Design review of the part built by this model. Coordinates are the model's own, in mm. Give positions to 0.01 mm unless a question says otherwise; leave off trailing zeros. Loops run counter-clockwise (first coordinate to the right, second up) from the corner with the lowest first, then second, coordinate; pieces in that order, holes last. Notation, with made-up numbers: (28.5, 55) - (69.5, 55) arc R8 cw to (69.5, 69) - close; hole circle Ø10 at (3, 44.25). An arc over 180 degrees is marked (long way). One line per item, written item: value. Start each with the question number.
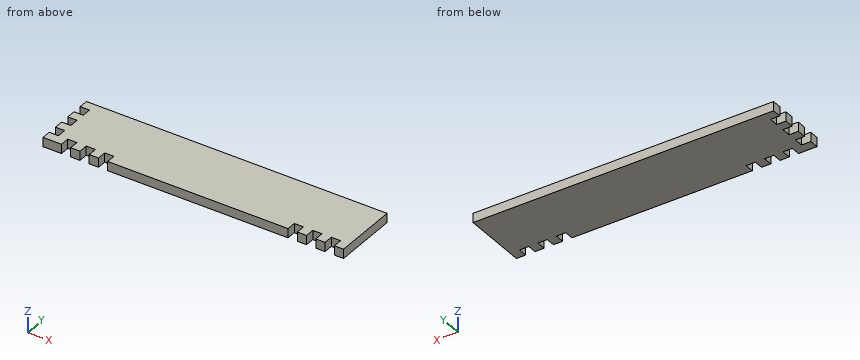
```python
from build123d import *

# Parameters (mm, degrees)
F0_W     = 412.75
F0_H     = 88.9
F1_DEPTH = 12.7
F2_W     = 12.7
F2_H     = 12.7
F3_DEPTH = 25.4
F4_W     = 12.7
F4_H     = 12.7
F5_DEPTH = 25.4
F6_W     = 12.7
F6_H     = 12.7
F7_DEPTH = 25.4


with BuildPart() as f1:
    # F0 (on Top) → F1 (new body)
    with BuildSketch(Plane.XY):
        with Locations((206.375, 44.45)):
            Rectangle(F0_W, F0_H)
    extrude(amount=F1_DEPTH)

    # F2 (on face) → F3 (cut)
    with BuildSketch(Plane.XY.offset(12.7)):
        with Locations((6.35, 19.05)):
            Rectangle(F2_W, F2_H)
        with Locations((6.35, 69.85)):
            Rectangle(F2_W, F2_H)
        with Locations((6.35, 44.45)):
            Rectangle(F2_W, F2_H)
    extrude(amount=-F3_DEPTH, mode=Mode.SUBTRACT)

    # F4 (on face) → F5 (cut)
    with BuildSketch(Plane.XY.offset(12.7)):
        with Locations((393.7, 6.35)):
            Rectangle(F4_W, F4_H)
        with Locations((368.3, 6.35)):
            Rectangle(F4_W, F4_H)
        with Locations((342.9, 6.35)):
            Rectangle(F4_W, F4_H)
    extrude(amount=-F5_DEPTH, mode=Mode.SUBTRACT)

    # F6 (on face) → F7 (cut)
    with BuildSketch(Plane.XY.offset(12.7)):
        with Locations((31.75, 6.35)):
            Rectangle(F6_W, F6_H)
        with Locations((57.15, 6.35)):
            Rectangle(F6_W, F6_H)
        with Locations((82.55, 6.35)):
            Rectangle(F6_W, F6_H)
    extrude(amount=-F7_DEPTH, mode=Mode.SUBTRACT)


solid = f1.part
```
(1) For pin 1 Ø6.5 at (y, z) = (71.5, 4.5) entering from -X, flat-tipped, find the tip position at first contact; note if it passes through.
(2) To check wall thickness, follow L1, parallel to Y at x = 59, z = 1.25; L2, parallel to X at y = 43, z = 12.25. State the ranges of each line that lie inside material, in increasing order. Write a range as from..to.
(3) Take a section at A-A on x = 365.5. State the section outline as (y, z) points, and give its area (3 significant figures).
Here are the results:
1. pin 1: x = 12.7
2. L1: 12.7..88.9
2. L2: 12.7..412.75
3. outline: (12.7, 0) - (88.9, 0) - (88.9, 12.7) - (12.7, 12.7) - close
3. area: 968 mm²
